Part print with two shaded views. Sizes in mm from the minimum x, y, z corner. Round coordinates to 2 decimals unless told otherwise and drop trailing zeros. Loops run counter-clockwise (first coordinate to the right, second up) from the corner with the lowest first, then second, coordinate; pieces in that order, holes last. Notation, with made-up numbers: M 17.5,-29 L 46.5,-29 A23 ccw 46.5,-8 Z; hole C 60.25,-24.5 d6. An arc over 180 degrees is marked long. Answer as CSV lines item,"result". Start each with the question number.
Item 1: Band-saw the part on C-C (y = 1.05). Give the cut face in (x, z), and give its area (3 significant figures).
Item 2: Drop flat-ended pins along their axis: pin 1 Ø10 at (x, z) = (5, 19) entering from +Y; pin 2 Ø1 at (y, z) = (1.5, 7.5) entering from -X. Give the stop position or say it passes through.
Item 3: Band-saw the part on A-A (z = 2.25). Give the cut face in (x, y).
Item 4: Mould opens along X. For the marked faces 1 and 2 say: pulls with the +X half, pulls with the -X half, needs draft (parallel to the pull), parting line crosses it, or undercut.
Item 5: Band-saw the part on D-D (z = 17.5). Give the cut face in (x, y), and give its area (3 significant figures).
Item 6: Band-saw the part on B-B (x = 24.75). Give the cut face in (y, z), and give its area (3 significant figures).
Item 7: Wall check: line 1 (Y direction, x = 2, z = 14.75); line 2 (Y direction, x = 12.75, z = 9.5); line 3 (X direction, y = 0.8, z = 19.5). Give the ranges that are in metal, low to high.
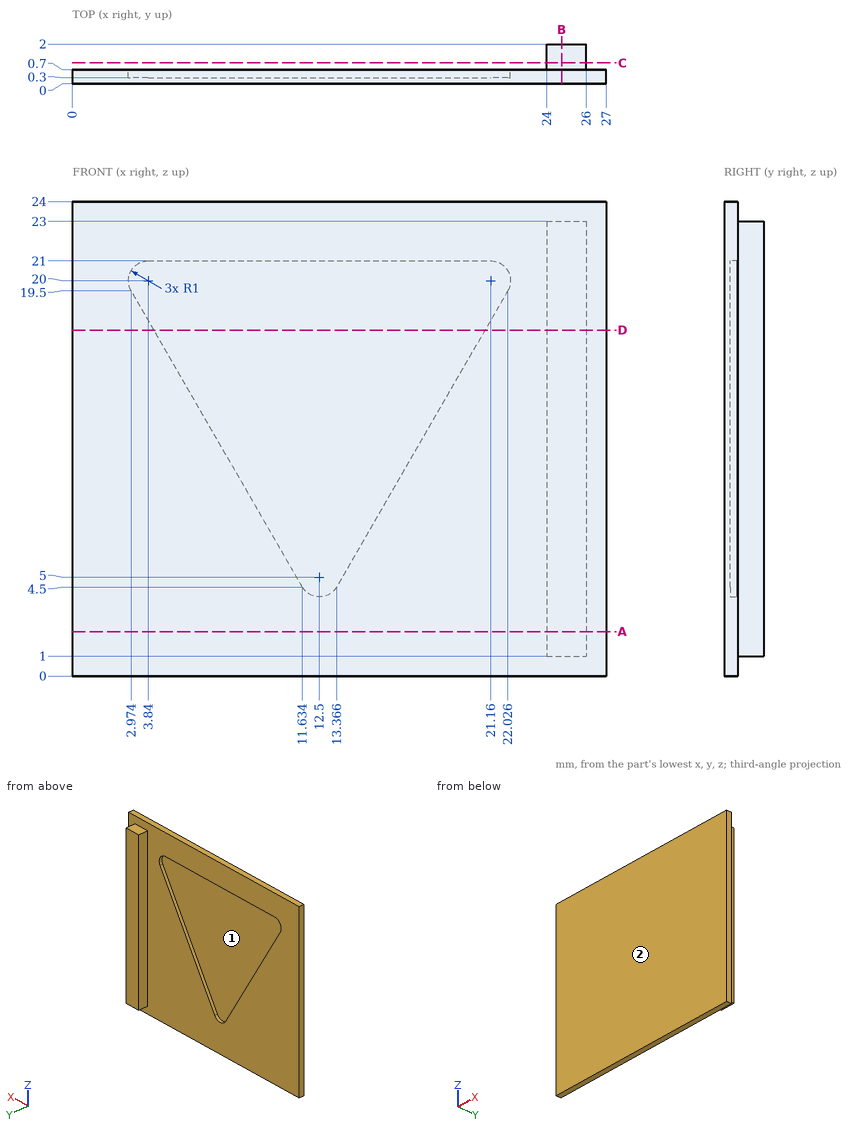
Answer block:
1,outline,"M 24,1 L 26,1 L 26,23 L 24,23 Z"
1,area,"44.0 mm^2"
2,pin 1,"stops at y = 0.7"
2,pin 2,"stops at x = 24"
3,outline,"M 0,0 L 27,0 L 27,0.7 L 26,0.7 L 26,2 L 24,2 L 24,0.7 L 0,0.7 Z"
4,face 1,"undercut"
4,face 2,"needs draft"
5,outline,"M 0,0 L 27,0 L 27,0.7 L 26,0.7 L 26,2 L 24,2 L 24,0.7 L 20.87,0.7 L 20.87,0.3 L 4.13,0.3 L 4.13,0.7 L 0,0.7 Z"
5,area,"14.8 mm^2"
6,outline,"M 0,0 L 0.7,0 L 0.7,1 L 2,1 L 2,23 L 0.7,23 L 0.7,24 L 0,24 Z"
6,area,"45.4 mm^2"
7,line 1,"y = 0 to 0.7"
7,line 2,"y = 0 to 0.3"
7,line 3,"x = 24 to 26"
